The figure shows three views and two pictorial views of one solid part (mm, origin at its lowest corner). Answer the questions. Give positions to 0.01 mm unless a question says otherwise; leave off trailing zeros. Order: outer loops, then holes, each group sorted by start corner. A loop starts at its lowest first (then second) coordinate and runs counter-clockwise, first axis right, second up. Notation, with made-up numbers: (66.5, -37.75) - (122.5, -37.75) arc R11 ccw to (122.5, -31.75) - close; hole circle Ø9 at (19.25, 16.25). An arc over 180 degrees is marked (long way). Use a Markdown table: item, result. Add a question column.
1. A cutting plane is placed at A-A on z = 32. Determine the outline of the cut face in (x, y), and give its area (3 significant figures).
2. For a pull along Y with two mould halves and no side action, classify the marked faces 1, 2 and 3 as released by +Y, released by -Y, zero draft, split by the parting line, or undercut.
3. Consider L1, parallel to Y at x = 79.5, z = 52.5; L2, parallel to Z at x = 90.5, y = 7.5 (1 decimal); L3, parallel to X at y = 27.5, z = 29 (1 decimal). Determine where each line is inside the solid, lowest interval first.
4. A cutting plane is placed at D-D on z = 71. Determine the outline of the cut face in (x, y), and give its area (3 significant figures).
5. Flat-ended cylindrical pins translate along their axes: P1, Ø12, axis at y = 5.5, z = 26.5, coming from the -X side; P2, Ø1.4, axis at x = 39.02, z = 13.36, coming from the +Y side; P3, Ø2, axis at y = 4, z = 78.5, coming from the +X side (1 decimal); P4, Ø1, axis at x = 138, y = 5.5, coming from the +Z side. Find the tip coordinate at first contact, or state that the pin passes through.
6. A cutting plane is placed at B-B on y = 29. State how many separate pieces and enclosed holes the cut face has, and give its area (3 significant figures).
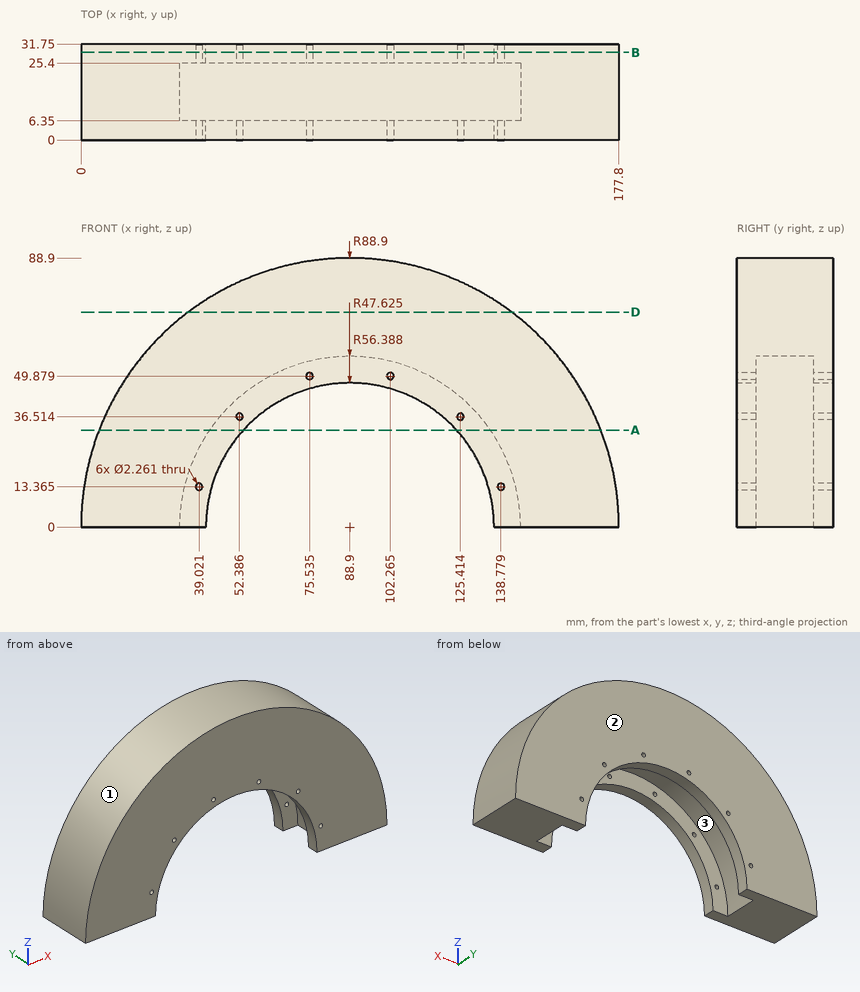
Output values:
| question | item | result |
|---|---|---|
| 1 | outline | (5.96, 0) - (53.63, 0) - (53.63, 6.35) - (42.47, 6.35) - (42.47, 25.4) - (53.63, 25.4) - (53.63, 31.75) - (5.96, 31.75) - close; (124.17, 0) - (171.84, 0) - (171.84, 31.75) - (124.17, 31.75) - (124.17, 25.4) - (135.33, 25.4) - (135.33, 6.35) - (124.17, 6.35) - close |
| 1 | area | 2,600 mm² |
| 2 | face 1 | zero draft |
| 2 | face 2 | released by +Y |
| 2 | face 3 | undercut |
| 3 | L1 | 0 to 6.35, 25.4 to 31.75 |
| 3 | L2 | 56.4 to 88.9 |
| 3 | L3 | 4.9 to 51.1, 126.7 to 172.9 |
| 4 | outline | (35.4, 0) - (142.4, 0) - (142.4, 31.75) - (35.4, 31.75) - close |
| 4 | area | 3,400 mm² |
| 5 | P1 | x = 2.4 |
| 5 | P2 | through |
| 5 | P3 | x = 132.5 |
| 5 | P4 | z = 74.44 |
| 6 | separate pieces | 1 |
| 6 | enclosed holes | 6 |
| 6 | area | 8,830 mm² |
